```python
from build123d import *

# Parameters (mm, degrees)
CHAMFER1_SIZE = 0.396875


with BuildPart() as part:
    # Sketch1 → Revolve1 (revolve)
    with BuildSketch(Plane(origin=(0, 0, 0), x_dir=(1, 0, 0), z_dir=(0, 1, 0))):
        with BuildLine():
            Line((0, 73.025), (0, -73.025))
            Line((0, -73.025), (6.35, -73.025))
            Line((6.35, -73.025), (6.35, -28.575))
            ThreePointArc((6.35, -28.575), (4.94058927, -26.499537373), (4.445, -24.040192948))
            Line((4.445, -24.040192948), (4.445, 24.040192948))
            ThreePointArc((4.445, 24.040192948), (4.94058927, 26.499537373), (6.35, 28.575))
            Line((6.35, 28.575), (6.35, 73.025))
            Line((6.35, 73.025), (0, 73.025))
        make_face()
    revolve(axis=Axis((0, 0, -73.025), (0, 0, 1)))

    # Chamfer1
    chamfer1_edges = [part.edges().sort_by_distance(p)[0] for p in [
        (-6.35, 0, 73.025),
        (-6.35, 0, -73.025),
    ]]
    chamfer(chamfer1_edges, length=CHAMFER1_SIZE)


solid = part.part
```
For this review, take the finished solid that the model builds, in its own axes (mm). Coordinates: 2 decimals unless noted, no trailing zeros. Write each loop counter-clockwise with the first axis right and the second up, starting at its lowest first coordinate (ties: lowest second). Pieces come first, ordered by that corner, then holes. Notation, with made-up numbers: (77, -23) - (128, -23) arc R23 cw to (128, -3) - close; hole circle Ø3 at (51, 5.25). An arc over 180 degrees is marked (long way). Put each result on its own line as item: value.
1. Add section C-C, the plane z = -10. Give the boundary of the cut face in (x, y) (3 decimals).
Values found:
outline: circle Ø8.89 at (0, 0)
2. Mouldability with a two-part tool opening along Z and no side actions: class faces 1 (the flat face through (0, 0, 73.025)), 2 (the cylindrical face through (-0.96, -4.34, -0.34)), 3 (the flat face through (0, 0, -73.025)) as released by +Z, released by -Z, zero draft, split by the parting line, or undercut.
Values found:
face 1: released by +Z
face 2: undercut
face 3: released by -Z
3. Add section A-A, the plane x = 0. Give the boundary of the cut face in (y, z) (3 decimals).
Values found:
outline: (-6.35, -72.628) - (-5.953, -73.025) - (5.953, -73.025) - (6.35, -72.628) - (6.35, -28.575) arc R6.35 cw to (4.445, -24.04) - (4.445, 24.04) arc R6.35 cw to (6.35, 28.575) - (6.35, 72.628) - (5.953, 73.025) - (-5.953, 73.025) - (-6.35, 72.628) - (-6.35, 28.575) arc R6.35 cw to (-4.445, 24.04) - (-4.445, -24.04) arc R6.35 cw to (-6.35, -28.575) - close
4. For pin 1 (5 mm diameter, centred on y = 0.5, z = 24, fed in from +X); pin 2 (1.5 mm diameter, centred on y = 2, z = 1, fed in from +X), all flat-tipped, find the tip position at first contact; note any pin that passes through.
Values found:
pin 1: x = 4.93
pin 2: x = 4.27
5. Add section D-D, the plane z = -51.5. Give the boundary of the cut face in (x, y).
Values found:
outline: circle Ø12.7 at (0, 0)
6. Wall thickness on probe 1 along Z at (x, y) = (-1.25, -5.5) (3 decimals); probe 2 along Z at (x, y) = (4, -3.5) (3 decimals); probe 3 along X at (y, z) = (5.25, -63.5): over which ranges is each line inside the solid? List them lowest first.
Values found:
probe 1: -73.025 to -27.748, 27.748 to 73.025
probe 2: -73.025 to -27.248, 27.248 to 73.025
probe 3: -3.57 to 3.57
